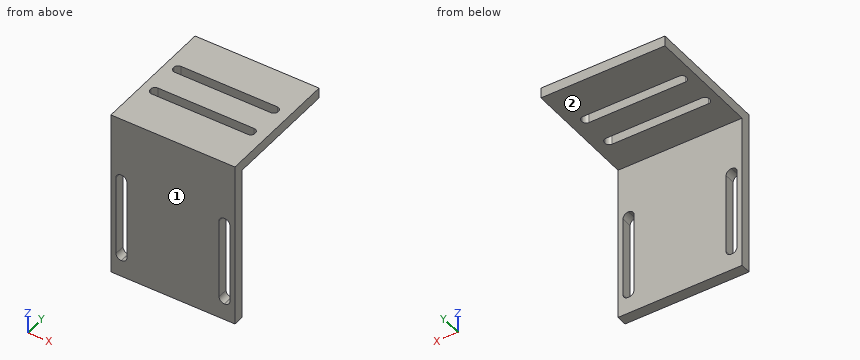
```python
from build123d import *

# Parameters (mm, degrees)
SKETCH1_W           = 37.592
SKETCH1_H           = 50.8
BOSS_EXTRUDE1_DEPTH = 3.175
SKETCH2_W           = 37.592
SKETCH2_H           = 3.175
BOSS_EXTRUDE2_DEPTH = 34.925
CUT_EXTRUDE1_REACH  = 52.8
CUT_EXTRUDE2_REACH  = 40.1


with BuildPart() as part:
    # Sketch1 → Boss-Extrude1 (new body)
    with BuildSketch(Plane(origin=(0, 0, 0), x_dir=(1, 0, 0), z_dir=(0, 1, 0))):
        Rectangle(SKETCH1_W, SKETCH1_H)
    extrude(amount=BOSS_EXTRUDE1_DEPTH)

    # Sketch2 → Boss-Extrude2 (add)
    with BuildSketch(Plane(origin=(0, 3.175, 0), x_dir=(1, 0, 0), z_dir=(0, 1, 0))):
        with Locations((0, -23.8125)):
            Rectangle(SKETCH2_W, SKETCH2_H)
    extrude(amount=BOSS_EXTRUDE2_DEPTH)

    # Sketch3 → Cut-Extrude1 (cut, up to next)
    with BuildSketch(Plane.XY.offset(25.4), mode=Mode.PRIVATE) as cut_extrude1_sk1:
        with BuildLine():
            Line((14.224, 12.7), (-14.986, 12.7))
            ThreePointArc((-14.986, 12.7), (-15.884025612, 13.071974388), (-16.256, 13.97))
            Line((-16.256, 13.97), (-16.256, 14.2748))
            ThreePointArc((-16.256, 14.2748), (-15.884025612, 15.172825612), (-14.986, 15.5448))
            Line((-14.986, 15.5448), (14.224, 15.5448))
            ThreePointArc((14.224, 15.5448), (15.122025612, 15.172825612), (15.494, 14.2748))
            Line((15.494, 14.2748), (15.494, 13.97))
            ThreePointArc((15.494, 13.97), (15.122025612, 13.071974388), (14.224, 12.7))
        make_face()
    cut_extrude1_tool1 = extrude(cut_extrude1_sk1.sketch, amount=-CUT_EXTRUDE1_REACH, mode=Mode.PRIVATE) & part.part
    add(cut_extrude1_tool1.solids().sort_by_distance((-0.381, 14.1224, 25.4))[0], mode=Mode.SUBTRACT)
    # Sketch3 → Cut-Extrude1 (cut, up to next)
    with BuildSketch(Plane.XY.offset(25.4), mode=Mode.PRIVATE) as cut_extrude1_sk2:
        with BuildLine():
            Line((-14.986, 23.1648), (14.224, 23.1648))
            ThreePointArc((14.224, 23.1648), (15.122025612, 23.536774388), (15.494, 24.4348))
            Line((15.494, 24.4348), (15.494, 24.7396))
            ThreePointArc((15.494, 24.7396), (15.122025612, 25.637625612), (14.224, 26.0096))
            Line((14.224, 26.0096), (-14.986, 26.0096))
            ThreePointArc((-14.986, 26.0096), (-15.884025612, 25.637625612), (-16.256, 24.7396))
            Line((-16.256, 24.7396), (-16.256, 24.4348))
            ThreePointArc((-16.256, 24.4348), (-15.884025612, 23.536774388), (-14.986, 23.1648))
        make_face()
    cut_extrude1_tool2 = extrude(cut_extrude1_sk2.sketch, amount=-CUT_EXTRUDE1_REACH, mode=Mode.PRIVATE) & part.part
    add(cut_extrude1_tool2.solids().sort_by_distance((-0.381, 24.5872, 25.4))[0], mode=Mode.SUBTRACT)

    # Sketch4 → Cut-Extrude2 (cut, up to next)
    with BuildSketch(Plane.XZ, mode=Mode.PRIVATE) as cut_extrude2_sk1:
        with BuildLine():
            Line((-15.5575, -20.32), (-15.6845, -20.32))
            ThreePointArc((-15.6845, -20.32), (-16.807032015, -19.855032015), (-17.272, -18.7325))
            Line((-17.272, -18.7325), (-17.272, 5.759956222))
            ThreePointArc((-17.272, 5.759956222), (-16.807032015, 6.882488237), (-15.6845, 7.347456222))
            Line((-15.6845, 7.347456222), (-15.5575, 7.347456222))
            ThreePointArc((-15.5575, 7.347456222), (-14.434967985, 6.882488237), (-13.97, 5.759956222))
            Line((-13.97, 5.759956222), (-13.97, -18.7325))
            ThreePointArc((-13.97, -18.7325), (-14.434967985, -19.855032015), (-15.5575, -20.32))
        make_face()
    cut_extrude2_tool1 = extrude(cut_extrude2_sk1.sketch, amount=-CUT_EXTRUDE2_REACH, mode=Mode.PRIVATE) & part.part
    add(cut_extrude2_tool1.solids().sort_by_distance((-15.621, 0, -6.486272))[0], mode=Mode.SUBTRACT)
    # Sketch4 → Cut-Extrude2 (cut, up to next)
    with BuildSketch(Plane.XZ, mode=Mode.PRIVATE) as cut_extrude2_sk2:
        with BuildLine():
            Line((15.6845, -20.32), (15.5575, -20.32))
            ThreePointArc((15.5575, -20.32), (14.434967985, -19.855032015), (13.97, -18.7325))
            Line((13.97, -18.7325), (13.97, 5.759956222))
            ThreePointArc((13.97, 5.759956222), (14.434967985, 6.882488237), (15.5575, 7.347456222))
            Line((15.5575, 7.347456222), (15.6845, 7.347456222))
            ThreePointArc((15.6845, 7.347456222), (16.807032015, 6.882488237), (17.272, 5.759956222))
            Line((17.272, 5.759956222), (17.272, -18.7325))
            ThreePointArc((17.272, -18.7325), (16.807032015, -19.855032015), (15.6845, -20.32))
        make_face()
    cut_extrude2_tool2 = extrude(cut_extrude2_sk2.sketch, amount=-CUT_EXTRUDE2_REACH, mode=Mode.PRIVATE) & part.part
    add(cut_extrude2_tool2.solids().sort_by_distance((15.621, 0, -6.486272))[0], mode=Mode.SUBTRACT)


solid = part.part
```
Could you check a few things on this model? Use its own coordinates, in mm. Face numbers are marked on the shaded views. A direction names the side the tool comes from. Round coordinates to 2 decimals unless told otherwise and drop trailing zeros. Write each loop counter-clockwise with the first axis right and the second up, starting at its lowest first coordinate (ties: lowest second). Pieces come first, ordered by that corner, then holes. Notation, with made-up numbers: M 23,11.25 L 28,11.25 A16 cw 28,17.25 Z; hole C 67,-6 d11. An arc over 180 degrees is marked long. Answer in a Markdown table with one row per item. Add a question column.
Q1. Imagine slicing it at B-B (x = 10.5). Please give me the cut outline in (y, z) (3 decimals).
Q2. Imagine slicing it at D-D (y = 36). Please give me the cut outline in (x, z) (3 decimals).
Q3. Imagine slicing it at C-C (z = -19.5). Please give me the cut outline in (x, y) (3 decimals).
Q4. Imagine slicing it at A-A (z = -14). Please give me the cut outline in (x, y) (3 decimals).
Q5. If I drill on line 1 (Y direction, x = -12, z = 22.5); line 2 (X direction, y = 3, z = -5.5); line 3 (X direction, y = 2, z = -19), over which ranges is the centre line in solid material (lowest first)? Write a range as from..to.
Q6. On a 3-axis mill with a long thin cutter (end or side, diameter ignored), from which of +Z, -Z, +X, -X, +Y, -Y can I reach the whole of each face in a straight line? I mean the marked faces 1 and 2. Say none if no direction works.
Q7. Will these pins go through, and if not, where does the flat tip stop? pin 1 Ø8 at (x, y) = (13.5, 28.5) entering from -Z (3 decimals); pin 2 Ø19 at (x, z) = (-3.5, -0.5) entering from +Y (3 decimals); pin 3 Ø2 at (x, y) = (8, 24.5) entering from -Z.
Values:
| question | item | result |
|---|---|---|
| 1 | outline | M 0,-25.4 L 3.175,-25.4 L 3.175,22.225 L 12.7,22.225 L 12.7,25.4 L 0,25.4 Z; M 15.545,22.225 L 23.165,22.225 L 23.165,25.4 L 15.545,25.4 Z; M 26.01,22.225 L 38.1,22.225 L 38.1,25.4 L 26.01,25.4 Z |
| 2 | outline | M -18.796,22.225 L 18.796,22.225 L 18.796,25.4 L -18.796,25.4 Z |
| 3 | outline | M -18.796,0 L -17.074,0 L -17.074,3.175 L -18.796,3.175 Z; M -14.168,0 L 14.168,0 L 14.168,3.175 L -14.168,3.175 Z; M 17.074,0 L 18.796,0 L 18.796,3.175 L 17.074,3.175 Z |
| 4 | outline | M -18.796,0 L -17.272,0 L -17.272,3.175 L -18.796,3.175 Z; M -13.97,0 L 13.97,0 L 13.97,3.175 L -13.97,3.175 Z; M 17.272,0 L 18.796,0 L 18.796,3.175 L 17.272,3.175 Z |
| 5 | line 1 | 0..12.7, 15.54..23.16, 26.01..38.1 |
| 5 | line 2 | -18.8..-17.27, -13.97..13.97, 17.27..18.8 |
| 5 | line 3 | -18.8..-17.25, -13.99..13.99, 17.25..18.8 |
| 6 | face 1 | +Z, -Z, +X, -X, -Y |
| 6 | face 2 | -Z, +X, -X, +Y |
| 7 | pin 1 | z = 22.225 |
| 7 | pin 2 | y = 3.175 |
| 7 | pin 3 | through |
